Can you work these out from the model? Positions are in its coordinate system, mm. A direction names the side the tool comes from. Round coordinates to 2 decimals unless told otherwise and drop trailing zeros. Loops run counter-clockwise (first coordinate to the right, second up) from the corner with the lowest first, then second, coordinate; pieces in that order, holes last. Notation, with made-up numbers: (-9.75, 17.5) -> (6.25, 17.5) arc R22 cw to (6.25, 36.5) -> close; hole circle Ø8 at (83, 73). An arc over 180 degrees is marked (long way). Write each question's results on one line, items separated by ' | '.
from build123d import *

# Parameters (mm, degrees)
SKETCH1_W           = 126
SKETCH1_H           = 60
BOSS_EXTRUDE1_DEPTH = 28
SKETCH2_W           = 106.5
SKETCH2_H           = 60
BOSS_EXTRUDE2_DEPTH = 6
SKETCH3_R           = 1.270837117
SKETCH3_R_2         = 10.401878768
SKETCH3_R_3         = 6.366682124
SKETCH3_W           = 2.541674233
SKETCH3_H           = 19.855616704
CUT_EXTRUDE1_DEPTH  = 1


with BuildPart() as part:
    # Sketch1 → Boss-Extrude1 (new body)
    with BuildSketch(Plane(origin=(0, 0, 0), x_dir=(1, 0, 0), z_dir=(0, 1, 0))):
        with Locations((63, 30)):
            Rectangle(SKETCH1_W, SKETCH1_H)
    extrude(amount=BOSS_EXTRUDE1_DEPTH)

    # Sketch2 → Boss-Extrude2 (add)
    with BuildSketch(Plane(origin=(0, 28, 0), x_dir=(1, 0, 0), z_dir=(0, 1, 0))):
        with Locations((53.25, 30)):
            Rectangle(SKETCH2_W, SKETCH2_H)
    extrude(amount=BOSS_EXTRUDE2_DEPTH)

    # Sketch3 → Cut-Extrude1 (cut)
    # profile 1 of 5: a face of its own
    with BuildSketch(Plane(origin=(0, 34, 0), x_dir=(1, 0, 0), z_dir=(0, 1, 0))):
        with Locations(Location((39.51710712, 40.365620358, 0), (0, 0, 270))):
            Circle(SKETCH3_R)
    # profile 2 of 5: a face of its own
    with BuildSketch(Plane(origin=(0, 34, 0), x_dir=(1, 0, 0), z_dir=(0, 1, 0))):
        with Locations(Location((86.125525447, 24.033278021, 0), (0, 0, 270))):
            Circle(SKETCH3_R_2)
        with Locations(Location((86.125525447, 24.033278021, 0), (0, 0, 270))):
            Circle(SKETCH3_R_3, mode=Mode.SUBTRACT)
    # profile 3 of 5: a face of its own
    with BuildSketch(Plane(origin=(0, 34, 0), x_dir=(1, 0, 0), z_dir=(0, 1, 0))):
        with BuildLine():
            Line((14.499134375, 40.429605669), (14.499134375, 14.579540085))
            Line((14.499134375, 14.579540085), (16.546664322, 14.579540085))
            Line((16.546664322, 14.579540085), (16.546664322, 29.680073446))
            ThreePointArc((16.546664322, 29.680073446), (27.232211234, 40.365620358), (16.546664322, 51.05116727))
            Line((16.546664322, 51.05116727), (14.499134375, 51.05116727))
            Line((14.499134375, 51.05116727), (14.499134375, 40.429605669))
        make_face()
        with BuildLine():
            Line((16.546664322, 48.080160925), (16.546664322, 32.651079791))
            ThreePointArc((16.546664322, 32.651079791), (24.26120489, 40.365620358), (16.546664322, 48.080160925))
        make_face(mode=Mode.SUBTRACT)
    # profile 4 of 5: a face of its own
    with BuildSketch(Plane(origin=(0, 34, 0), x_dir=(1, 0, 0), z_dir=(0, 1, 0))):
        with Locations((39.517107119, 24.507348437)):
            Rectangle(SKETCH3_W, SKETCH3_H)
    # profile 5 of 5: a face of its own
    with BuildSketch(Plane(origin=(0, 34, 0), x_dir=(1, 0, 0), z_dir=(0, 1, 0))):
        with BuildLine():
            Line((67.74148212, 32.262991734), (66.622002756, 30.534452251))
            ThreePointArc((66.622002756, 30.534452251), (54.221440679, 23.691888532), (67.166075127, 17.944623349))
            Line((67.166075127, 17.944623349), (68.322309862, 16.231868944))
            ThreePointArc((68.322309862, 16.231868944), (52.161989467, 23.672443665), (67.74148212, 32.262991734))
        make_face()
    extrude(amount=-CUT_EXTRUDE1_DEPTH, mode=Mode.SUBTRACT)


solid = part.part
1. If we section it at D-D (z = -22): List the corners of the cut face in (x, y) for me.
Final values:
outline: (0, 0) -> (126, 0) -> (126, 28) -> (106.5, 28) -> (106.5, 34) -> (96.33, 34) -> (96.33, 33) -> (92.16, 33) -> (92.16, 34) -> (80.09, 34) -> (80.09, 33) -> (75.92, 33) -> (75.92, 34) -> (54.48, 34) -> (54.48, 33) -> (52.37, 33) -> (52.37, 34) -> (40.79, 34) -> (40.79, 33) -> (38.25, 33) -> (38.25, 34) -> (16.55, 34) -> (16.55, 33) -> (14.5, 33) -> (14.5, 34) -> (0, 34) -> close
2. If we section it at C-C (y = 30.5): List the corners of the cut face in (x, z) for me.
Final values:
outline: (0, -60) -> (106.5, -60) -> (106.5, 0) -> (0, 0) -> close
3. We'd pull the mould along X, two halves only. Please class faces 4 (the face through (54, 33, -23)), 5 (the face through (54.215, 33.507, -23.937)), 6 (the face through (86, 34, -24)), 7 (the face through (106.5, 31, -30)): pulls with the +X half, pulls with the -X half, needs draft (parallel to the pull), parting line crosses it, or undercut.
Final values:
face 4: undercut | face 5: undercut | face 6: needs draft | face 7: pulls with the +X half
4. If we section it at B-B (x = 113): List the corners of the cut face in (y, z) for me, then the cut area to 3 significant figures.
Final values:
outline: (0, -60) -> (28, -60) -> (28, 0) -> (0, 0) -> close | area: 1,680 mm2
5. On a 3-axis mill with a long thin cutter (end or side, diameter ignored), from which of +Z, -Z, +X, -X, +Y, -Y can I reach the whole of each face in a straight line? I mean faces 1 (the face through (62, 0, -30)), 2 (the face through (116, 28, -30)), 3 (the face through (94.896, 33.507, -18.441)). Say none if no direction works.
Final values:
face 1: +Z, -Z, +X, -X, -Y | face 2: +Z, -Z, +X, +Y | face 3: +Y
6. Please list where these lines run through material, in increasing order: line 1 (Y direction, x = 16, z = -19); line 2 (X direction, y = 30, z = -26); line 3 (Y direction, x = 109.5, z = -18). Write a range as from..to.
Final values:
line 1: 0..33 | line 2: 0..106.5 | line 3: 0..28
7. If we section it at A-A (z = -5): List the corners of the cut face in (x, y) for me.
Final values:
outline: (0, 0) -> (126, 0) -> (126, 28) -> (106.5, 28) -> (106.5, 34) -> (0, 34) -> close
8. Will these pins go through, and if not, where does the flat tip stop? pin 1 (3 mm diameter, centred on x = 40, z = -40, fed in from +Y); pin 2 (5 mm diameter, centred on y = 32.5, z = -29.5, fed in from +X); pin 3 (1.5 mm diameter, centred on x = 39.52, z = -40.37, fed in from +Y); pin 4 (10 mm diameter, centred on x = 116.5, z = -29.5, fed in from +Y).
Final values:
pin 1: y = 34 | pin 2: x = 106.5 | pin 3: y = 33 | pin 4: y = 28
